For this review, use the dimensioned drawing (mm, ordinates from the lowest corner) and the shaded views. A direction names the side the tool comes from. Round coordinates to 2 decimals unless told otherwise and drop trailing zeros. Order: outer loops, then holes, each group sorted by start corner. A loop starts at its lowest first (then second) coordinate and runs counter-clockwise, first axis right, second up. Notation, with made-up numbers: (4.5, 63.25) - (21.5, 63.25) arc R25 cw to (21.5, 91.25) - close; hole circle Ø4 at (71.25, 51). An arc over 180 degrees is marked (long way). Use CSV: the item, a comma, the result in double quotes. Start each with the question number.
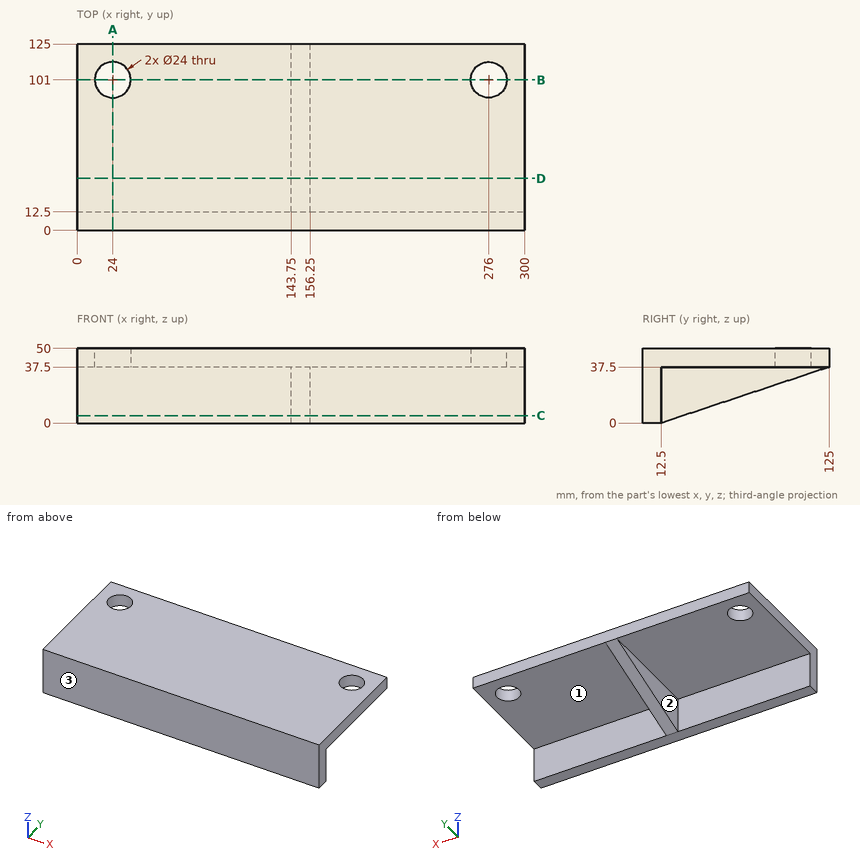
Q1. For L1, parallel to Y at x = 276, z = 41.25; L2, parallel to Z at x = 117.5, y = 107.5; L3, parallel to Y at x = 167, z = 4, list the stretches that pass through material, from the lowest coordinate up. Write a range as [from, to].
Q2. Take a section at C-C (z = 5). State the section outline as (x, y) points, plus the area to 3 significant figures.
Q3. Clearance check with flat-ended pins moving along their axes: pin 1 (19 mm diameter, centred on x = 276, y = 101, fed in from +Z) (1 decimal); pin 2 (12 mm diameter, centred on x = 57, z = 18, fed in from +Y); pin 3 (6 mm diameter, centred on x = 145, y = 19.5, fed in from -Z). State where each tip first meets the part, or that it passes through.
Q4. Take a section at D-D (y = 35). State the section outline as (x, z) points.
Q5. Tool access review of the marked faces 1, 2 and 3: name each direction out of +Z, -Z, +X, -X, +Y, -Y from which nothing blocks a thin tool from reaching the whole face with its end or side.
Q6. Take a section at B-B (y = 101). State the section outline as (x, z) points.
Q7. Take a section at A-A (x = 24). State the section outline as (y, z) points.
Findings below:
1,L1,"y = [0, 89], [113, 125]"
1,L2,"z = [37.5, 50]"
1,L3,"y = [0, 12.5]"
2,outline,"(0, 0) - (300, 0) - (300, 12.5) - (156.25, 12.5) - (156.25, 27.5) - (143.75, 27.5) - (143.75, 12.5) - (0, 12.5) - close"
2,area,"3,940 mm^2"
3,pin 1,"passes through"
3,pin 2,"stops at y = 12.5"
3,pin 3,"stops at z = 1.33"
4,outline,"(0, 37.5) - (143.75, 37.5) - (143.75, 7.5) - (156.25, 7.5) - (156.25, 37.5) - (300, 37.5) - (300, 50) - (0, 50) - close"
5,face 1,"-Z, +X, +Y"
5,face 2,"-Z, -X, +Y"
5,face 3,"+Z, -Z, +X, -X, -Y"
6,outline,"(0, 37.5) - (12, 37.5) - (12, 50) - (0, 50) - close; (36, 37.5) - (143.75, 37.5) - (143.75, 29.5) - (156.25, 29.5) - (156.25, 37.5) - (264, 37.5) - (264, 50) - (36, 50) - close; (288, 37.5) - (300, 37.5) - (300, 50) - (288, 50) - close"
7,outline,"(0, 0) - (12.5, 0) - (12.5, 37.5) - (89, 37.5) - (89, 50) - (0, 50) - close; (113, 37.5) - (125, 37.5) - (125, 50) - (113, 50) - close"
